Verification items for the finished model (mm, model axes). A direction names the side the tool comes from. Round coordinates to 2 decimals unless told otherwise and drop trailing zeros. Loops run counter-clockwise (first coordinate to the right, second up) from the corner with the lowest first, then second, coordinate; pieces in that order, holes last. Notation, with made-up numbers: (6.5, 56) -> (15.5, 56) arc R19 cw to (15.5, 60) -> close; hole circle Ø10 at (-15, -39). An arc over 180 degrees is marked (long way). Write item = value, one per line. Start each with the question number.
```python
from build123d import *

# Parameters (mm, degrees)
EXTRUDE_THIN1_DEPTH = 38
CUT_EXTRUDE1_DEPTH  = 4
FILLET1_R           = 3.5
FILLET2_R           = 3.5
CUT_EXTRUDE2_DEPTH  = 4


with BuildPart() as part:
    # Sketch2 → Extrude-Thin1 (new body)
    with BuildSketch(Plane(origin=(0, 0, 0), x_dir=(0, 0, -1), z_dir=(1, 0, 0))):
        Polygon((-63, 0), (0, 0), (0, 26.25), (-3, 26.25), (-3, 3), (-63, 3), align=None)
    extrude(amount=-EXTRUDE_THIN1_DEPTH)

    # Sketch3 → Cut-Extrude1 (cut, through all)
    with BuildSketch(Plane.XY.offset(3)):
        with BuildLine():
            Line((-29.5, 11.5), (-22.5, 11.5))
            ThreePointArc((-22.5, 11.5), (-19.5, 8.5), (-22.5, 5.5))
            Line((-22.5, 5.5), (-29.5, 5.5))
            ThreePointArc((-29.5, 5.5), (-32.5, 8.5), (-29.5, 11.5))
        make_face()
        with BuildLine():
            Line((-15.5, 23.75), (-8.5, 23.75))
            ThreePointArc((-8.5, 23.75), (-5.5, 20.75), (-8.5, 17.75))
            Line((-8.5, 17.75), (-15.5, 17.75))
            ThreePointArc((-15.5, 17.75), (-18.5, 20.75), (-15.5, 23.75))
        make_face()
    extrude(amount=-CUT_EXTRUDE1_DEPTH, mode=Mode.SUBTRACT)

    # Fillet1
    fillet1_edges = [part.edges().sort_by_distance(p)[0] for p in [
        (-38, 26.25, 1.5),
    ]]
    fillet(fillet1_edges, radius=FILLET1_R)

    # Fillet2
    fillet2_edges = [part.edges().sort_by_distance(p)[0] for p in [
        (0, 26.25, 1.5),
    ]]
    fillet(fillet2_edges, radius=FILLET2_R)

    # Sketch4 → Cut-Extrude2 (cut, through all)
    with BuildSketch(Plane(origin=(0, 3, 0), x_dir=(1, 0, 0), z_dir=(0, 1, 0))):
        with BuildLine():
            Line((-33.5, -23.5), (-33.5, -42.5))
            ThreePointArc((-33.5, -42.5), (-19, -57), (-4.5, -42.5))
            Line((-4.5, -42.5), (-4.5, -23.5))
            ThreePointArc((-4.5, -23.5), (-19, -9), (-33.5, -23.5))
        make_face()
        with BuildLine():
            Line((0, -63), (0, -42.5))
            ThreePointArc((0, -42.5), (-19, -61.5), (-38, -42.5))
            Line((-38, -42.5), (-38, -63))
            Line((-38, -63), (0, -63))
        make_face()
    extrude(amount=-CUT_EXTRUDE2_DEPTH, mode=Mode.SUBTRACT)


solid = part.part
```
(1) Depth check by flat-ended pin: pin 1 Ø5 at (x, z) = (-23, 52) entering from +Y; pin 2 Ø19 at (x, z) = (-10.5, 46.5) entering from +Y; pin 3 Ø6 at (y, z) = (3.5, 47) entering from +X. Enter the tip coordinate at first touch or a pass-through.
(2) Draft check along X on faces 1 (the flat face through (-26, 11.5, 2)), 2 (the cylindrical face through (-19, 2, 57)), 3 (the flat face through (-19, 26.25, 1)), 4 (the cylindrical face through (-37, 25.2, 1.5)). Enter one of: +X half, -X half, draft (parallel to the pull), parting line (faces both ways), or undercut.
(3) Section check A-A on y = 8.5. Enter the section's corners in (x, z).
(4) Access from +Z, -Z, +X, -X, +Y, -Y to the whole of each face (thin tool, end or side, straight path). Record for faces 5 (the cylindrical face through (-19, 2, 9)), 6 (the flat face through (-19, 13, 0)), 7 (the cylindrical face through (-32.5, 8.4, 1.5)), 8 (the flat face through (-36, 3, 25)).
(5) Section check D-D on y = 12.75. Enter the section's corners in (x, z).
(6) Section check C-C on x = -27.5. Enter the section's corners in (y, z).
(7) Scan lines: line 1 (Y direction, x = -24.5, z = 7); line 2 (X direction, y = 2.25, z = 52). Record each from-to range of solid material in increasing order. Write a range as [from, to].
(8) Section check B-B on z = 31.5. Enter the section's corners in (x, y), then the cut area to 3 significant figures.
Computed values:
q1.pin_1 = through
q1.pin_2 = 3
q1.pin_3 = -0.06
q2.face_1 = undercut
q2.face_2 = undercut
q2.face_3 = draft
q2.face_4 = -X half
q3.outline = (-38, 0) -> (-32.5, 0) -> (-32.5, 3) -> (-38, 3) -> close; (-19.5, 0) -> (0, 0) -> (0, 3) -> (-19.5, 3) -> close
q4.face_5 = +Y, -Y
q4.face_6 = -Z, +X, -X, +Y, -Y
q4.face_7 = +Z, -Z
q4.face_8 = +Z, +X, -X, +Y
q5.outline = (-38, 0) -> (0, 0) -> (0, 3) -> (-38, 3) -> close
q6.outline = (0, 0) -> (5.5, 0) -> (5.5, 3) -> (3, 3) -> (3, 11.75) -> (0, 11.75) -> close; (0, 54.25) -> (3, 54.25) -> (3, 59.49) -> (0, 59.49) -> close; (11.5, 0) -> (26.25, 0) -> (26.25, 3) -> (11.5, 3) -> close
q7.line_1 = [0, 3]
q7.line_2 = [-35.45, -29.95], [-8.05, -2.55]
q8.outline = (-38, 0) -> (-33.5, 0) -> (-33.5, 3) -> (-38, 3) -> close; (-4.5, 0) -> (0, 0) -> (0, 3) -> (-4.5, 3) -> close
q8.area = 27.0 mm²
